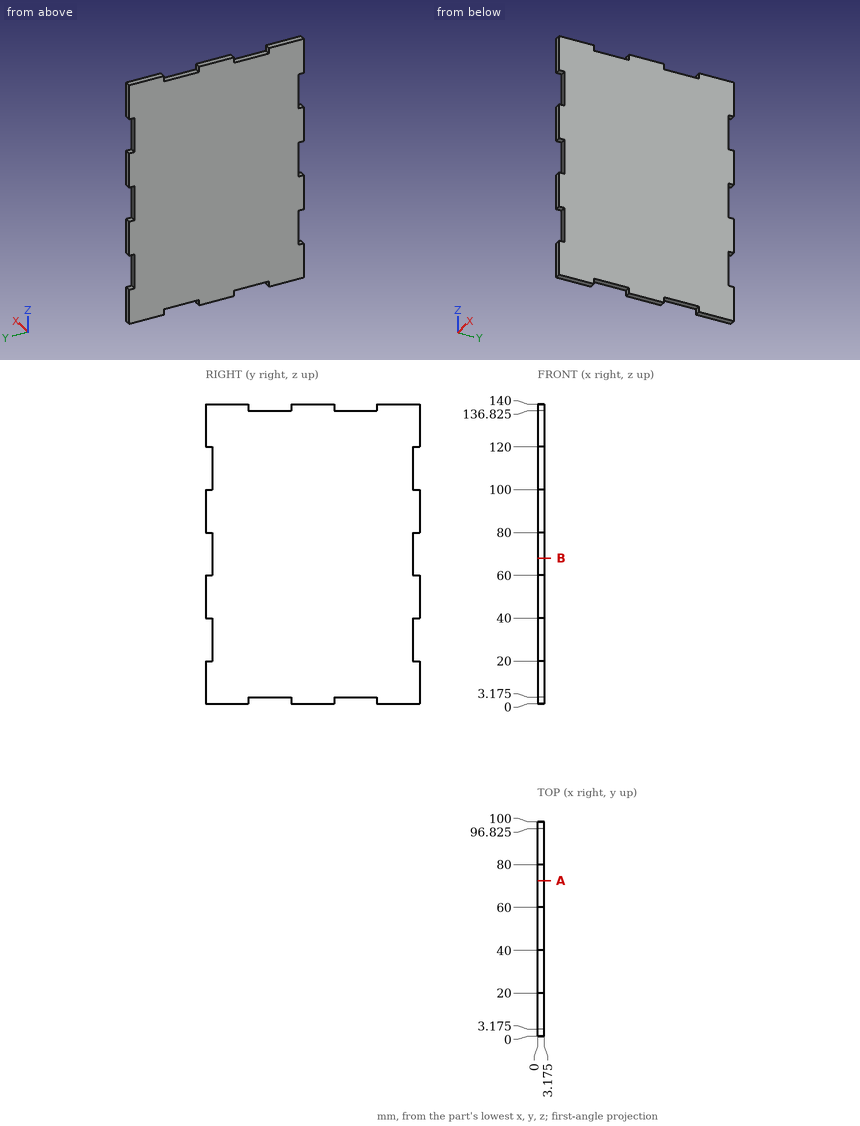
Can you work these out from the drawing? Everything is in mm from the part's minimum corner. Give positions to 0.01 mm unless a question says otherwise; leave off trailing zeros. Loops run counter-clockwise (first coordinate to the right, second up) from the corner with the lowest first, then second, coordinate; pieces in that order, holes last. Notation, with made-up numbers: (16, 58.25) -> (68, 58.25) arc R18 ccw to (68, 70.25) -> close; hole circle Ø2 at (29, 62.25). An arc over 180 degrees is marked (long way). Put each result on its own line as item: value.
(1) Imagine slicing it at A-A on y = 72.5. Write out the boundary of the cut face in (x, z) (3 decimals), plus the area to 3 significant figures.
Computed:
outline: (0, 3.175) -> (3.175, 3.175) -> (3.175, 136.825) -> (0, 136.825) -> close
area: 424 mm^2
(2) Imagine slicing it at B-B on z = 68. Write out the boundary of the cut face in (x, y) (3 decimals), plus the area to 3 significant figures.
Computed:
outline: (0, 3.175) -> (3.175, 3.175) -> (3.175, 96.825) -> (0, 96.825) -> close
area: 297 mm^2
(3) Please list where these lines run through material, in increasing order: probe 1 along Z at (x, y) = (0.65, 65) (3 decimals); probe 2 along Y at (x, z) = (1, 107.5) (3 decimals). Write a range as [from, to].
Computed:
probe 1: [3.175, 136.825]
probe 2: [3.175, 96.825]
(4) I'm going to push flat-ended pins straight in: pin 1 Ø1.6 at (x, z) = (2.5, 70) entering from -Y (3 decimals); pin 2 Ø1 at (x, z) = (1.5, 113.5) entering from +Y (3 decimals); pin 3 Ø1 at (x, y) = (2.5, 61.5) entering from -Z (3 decimals). Where does each tip first touch, or does it pass through?
Computed:
pin 1: y = 3.175
pin 2: y = 96.825
pin 3: z = 3.175
